from build123d import *

# Parameters (mm, degrees)
SKETCH_1_W                  = 76
SKETCH_1_H                  = 76
EXTRUDE_1_DEPTH             = 2
SKETCH_2_R                  = 1.6
CUT_EXTRUDE_1_DEPTH         = 2
PATTERN_LINEAR_1_COUNT      = 2
PATTERN_LINEAR_1_PITCH      = 60
PATTERN_LINEAR_1_COUNT_DIR2 = 2
PATTERN_LINEAR_1_PITCH_DIR2 = 60


with BuildPart() as part:
    # 草图1 → 凸台-拉伸1 (new body)
    with BuildSketch(Plane(origin=(0, 0, 0), x_dir=(1, 0, 0), z_dir=(0, 1, 0))):
        Rectangle(SKETCH_1_W, SKETCH_1_H)
    extrude(amount=EXTRUDE_1_DEPTH)

    # 草图2 → 切除-拉伸1 (cut)
    with BuildSketch(Plane(origin=(0, 2, 0), x_dir=(1, 0, 0), z_dir=(0, 1, 0))):
        with Locations(Location((-30, 30, 0), (0, 0, 270))):
            Circle(SKETCH_2_R)
    cut_extrude_1 = extrude(amount=-CUT_EXTRUDE_1_DEPTH, mode=Mode.SUBTRACT)

    # 阵列(线性)1: Cut-Extrude 1 2 × 2
    with Locations(*[(i * PATTERN_LINEAR_1_PITCH, 0, j * PATTERN_LINEAR_1_PITCH_DIR2) for i in range(PATTERN_LINEAR_1_COUNT) for j in range(PATTERN_LINEAR_1_COUNT_DIR2) if (i, j) != (0, 0)]):
        add(cut_extrude_1, mode=Mode.SUBTRACT)


solid = part.part
Can you work these out from the model? Positions are in its coordinate system, mm. Coordinates: 2 decimals unless noted, no trailing zeros. Loops run counter-clockwise (first coordinate to the right, second up) from the corner with the lowest first, then second, coordinate; pieces in that order, holes last. Notation, with made-up numbers: (-6, 48) - (1, 48) arc R37 ccw to (1, 84) - close; hole circle Ø7 at (67.25, 45). An arc over 180 degrees is marked (long way). Answer as a JSON object with one key per item and string values. Group by question number.
Item 1: If I drill on L1, parallel to X at y = 0.7, z = -30; L2, parallel to Z at x = 29, y = 1.85, over which ranges is the centre line in solid material (lowest first)? Write a range as from..to.
Item 2: If we section it at B-B (z = -30): List the corners of the cut face in (x, y) for me, plus the area to 3 significant figures.
Item 3: If we mould it in two halves opening along X, with no side actions, what happens to faces 1 (the face through (-38, 1, 1)), 2 (the face through (38, 1, 1)), 3 (the face through (31.08, 1.01, 28.82))? For each: released by +X, released by -X, zero draft, split by the parting line, or undercut.
Item 4: For pin 1 (2 mm diameter, centred on x = 2.5, z = -17.5, fed in from -Y); pin 2 (2.5 mm diameter, centred on x = 30, z = 30, fed in from +Y), each with a flat end and sliding along its axis, tell me the tip position at first contact or that it passes through.
Item 5: If we section it at A-A (x = 30): List the corners of the cut face in (y, z) for me.
Returned:
{
 "1": {"L1": "x = -38..-31.6, -28.4..28.4, 31.6..38", "L2": "z = -38..-31.25, -28.75..28.75, 31.25..38"},
 "2": {"outline": "(-38, 0) - (-31.6, 0) - (-31.6, 2) - (-38, 2) - close; (-28.4, 0) - (28.4, 0) - (28.4, 2) - (-28.4, 2) - close; (31.6, 0) - (38, 0) - (38, 2) - (31.6, 2) - close", "area": "139 mm²"},
 "3": {"face 1": "released by -X", "face 2": "released by +X", "face 3": "undercut"},
 "4": {"pin 1": "stops at y = 0", "pin 2": "passes through"},
 "5": {"outline": "(0, -38) - (2, -38) - (2, -31.6) - (0, -31.6) - close; (0, -28.4) - (2, -28.4) - (2, 28.4) - (0, 28.4) - close; (0, 31.6) - (2, 31.6) - (2, 38) - (0, 38) - close"}
}
